Autodesk Fusion 360 part; units mm, degrees
sketch "Boceto1" plane through (0, 0, 0) normal (0, 0, 1) x (1, 0, 0)
  circle A0 centre (0, 0) radius 29.2
  circle A1 centre (0, 23.3) radius 2.8
  circle A2 centre (-20.1784, 11.65) radius 2.8
  circle A3 centre (-20.1784, -11.65) radius 2.8
  circle A4 centre (0, -23.3) radius 2.8
  circle A5 centre (20.1784, -11.65) radius 2.8
  circle A6 centre (20.1784, 11.65) radius 2.8
  dimension "d1" = 58.4
  dimension "d2" = 5.6
  dimension "d4" = 360
  dimension "d14" = 23.3
extrude "Extruir1" add sketch "Boceto1" against normal blind 7
sketch "Boceto2" plane through (0, 0, 0) normal (0, 0, 1) x (-1, 0, 0)
  circle A0 centre (0, -23.3) radius 2.8
  circle A1 centre (20.1784, 11.65) radius 2.8
  circle A2 centre (20.1784, -11.65) radius 2.8
  circle A3 centre (0, 23.3) radius 2.8
  circle A4 centre (-20.1784, 11.65) radius 2.8
  circle A5 centre (-20.1784, -11.65) radius 2.8
  circle A6 centre (0, 0) radius 29.2
  circle A7 centre (0, 0) radius 6
  dimension "d7" = 12
extrude "Extruir2" add sketch "Boceto2" along normal blind 51 contours A7
sketch "Boceto3" plane through (0, 0, 51) normal (0, 0, 1) x (-1, 0, 0)
  circle A0 centre (0, 0) radius 6
  circle A1 centre (0, 0) radius 3.85
  dimension "d10" = 7.7
extrude "Extruir3" add sketch "Boceto3" along normal blind 10 contours A1
sketch "Boceto4" plane through (0, 0, 0) normal (0, 0, 1) x (-1, 0, 0)
  circle A0 centre (0, 0) radius 6
  circle A1 centre (0, -23.3) radius 2.8
  circle A2 centre (20.1784, 11.65) radius 2.8
  circle A3 centre (20.1784, -11.65) radius 2.8
  circle A4 centre (0, 23.3) radius 2.8
  circle A5 centre (-20.1784, 11.65) radius 2.8
  circle A6 centre (-20.1784, -11.65) radius 2.8
  circle A7 centre (0, 0) radius 29.2
  circle A8 centre (0, 0) radius 20.3
  dimension "d13" = 40.6
sketch "Boceto5" plane through (0, 0, 0) normal (0, 1, 0) x (1, 0, 0)
fillet "Empalme1" radius 12 1 edges at (5.594, -2.1697, 0)
sketch "Boceto6" plane through (0, 0, -7) normal (0, 0, -1) x (1, 0, 0)
  circle A0 centre (0, -23.3) radius 2.8
  circle A1 centre (-20.1784, -11.65) radius 2.8
  circle A2 centre (-20.1784, 11.65) radius 2.8
  circle A3 centre (0, 23.3) radius 2.8
  circle A4 centre (20.1784, 11.65) radius 2.8
  circle A5 centre (20.1784, -11.65) radius 2.8
  circle A6 centre (0, 0) radius 29.2
  circle A7 centre (0, 0) radius 6
  dimension "d17" = 12
extrude "Extruir4" add sketch "Boceto6" along normal blind 20 contours A7
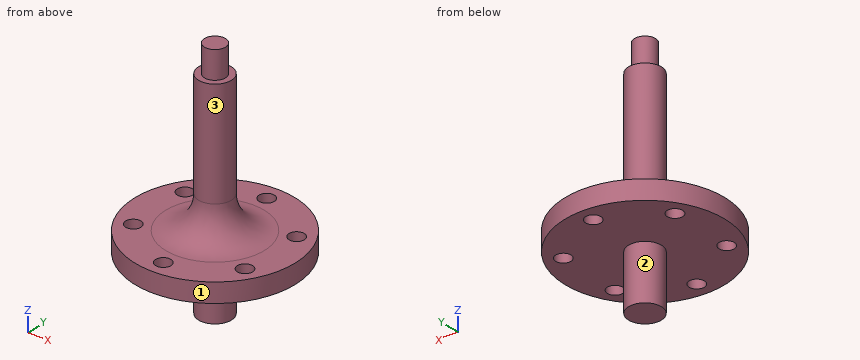
Could you check a few things on this model? Use its own coordinates, in mm. Face numbers are marked on the shaded views. A direction names the side the tool comes from. Give positions to 0.01 mm unless a question says otherwise; leave off trailing zeros. Write each loop counter-clockwise with the first axis right and the second up, starting at its lowest first coordinate (ties: lowest second). Pieces come first, ordered by that corner, then holes. Notation, with made-up numbers: (-38.5, -4) -> (-27.5, -4) arc R23 ccw to (-27.5, 14) -> close; hole circle Ø11 at (70.25, -31). An arc over 180 degrees is marked (long way). Write each question's results on one line, items separated by ' | '.
1. I need wall thicknesses on L1, parallel to Y at x = 0, z = -2.25; L2, parallel to X at y = -23, z = -2; L3, parallel to Z at x = 19, y = 0.5. Which ranges of each line are inside material? Lowest first, please.
Check sheet entries:
L1: y = -29.2 to -26.1, -20.5 to 20.5, 26.1 to 29.2 | L2: x = -17.99 to -2.78, 2.78 to 17.99 | L3: z = -7 to 0
2. Will these pins go through, and if not, where does the flat tip stop? pin 1 Ø3.5 at (x, y) = (0, 23.3) entering from +Z; pin 2 Ø4 at (x, y) = (14.5, 7.5) entering from +Z; pin 3 Ø9 at (x, y) = (-20.18, 11.65) entering from +Z; pin 4 Ø6.5 at (x, y) = (0, -23.3) entering from -Z.
Check sheet entries:
pin 1: passes through | pin 2: stops at z = 0.58 | pin 3: stops at z = 0 | pin 4: stops at z = -7
3. I want a section at B-B, the plane z = -1. Write out the boundary of the cut face in (x, y).
Check sheet entries:
outline: circle Ø58.4 at (0, 0); hole circle Ø5.6 at (-20.18, -11.65); hole circle Ø5.6 at (-20.18, 11.65); hole circle Ø5.6 at (0, -23.3); hole circle Ø5.6 at (0, 23.3); hole circle Ø5.6 at (20.18, -11.65); hole circle Ø5.6 at (20.18, 11.65)
4. I want a section at C-C, the plane y = -23.3. Write out the boundary of the cut face in (x, z), then the cut area to 3 significant figures.
Check sheet entries:
outline: (-17.6, -7) -> (-2.8, -7) -> (-2.8, 0) -> (-17.6, 0) -> close; (2.8, -7) -> (17.6, -7) -> (17.6, 0) -> (2.8, 0) -> close | area: 207 mm²
5. On a 3-axis mill with a long thin cutter (end or side, diameter ignored), from which of +Z, -Z, +X, -X, +Y, -Y can I reach the whole of each face in a straight line? I mean the marked faces 1, 2 and 3. Say none if no direction works.
Check sheet entries:
face 1: +Z, -Z | face 2: -Z | face 3: +Z
6. I want a section at D-D, the plane y = 0. Write out the boundary of the cut face in (x, z), then the cut area to 3 significant figures.
Check sheet entries:
outline: (-29.2, -7) -> (-6, -7) -> (-6, -27) -> (6, -27) -> (6, -7) -> (29.2, -7) -> (29.2, 0) -> (18, 0) arc R12 cw to (6, 12) -> (6, 51) -> (3.85, 51) -> (3.85, 61) -> (-3.85, 61) -> (-3.85, 51) -> (-6, 51) -> (-6, 12) arc R12 cw to (-18, 0) -> (-29.2, 0) -> close | area: 1,400 mm²
7. I want a section at A-A, the plane x = 0. Write out the boundary of the cut face in (y, z).
Check sheet entries:
outline: (-29.2, -7) -> (-26.1, -7) -> (-26.1, 0) -> (-29.2, 0) -> close; (-20.5, -7) -> (-6, -7) -> (-6, -27) -> (6, -27) -> (6, -7) -> (20.5, -7) -> (20.5, 0) -> (18, 0) arc R12 cw to (6, 12) -> (6, 51) -> (3.85, 51) -> (3.85, 61) -> (-3.85, 61) -> (-3.85, 51) -> (-6, 51) -> (-6, 12) arc R12 cw to (-18, 0) -> (-20.5, 0) -> close; (26.1, -7) -> (29.2, -7) -> (29.2, 0) -> (26.1, 0) -> close
